Geometry check sheet. Reference: the model listing, model coordinates, mm. Give positions to 0.01 mm unless a question says otherwise; leave off trailing zeros. Loops run counter-clockwise (first coordinate to the right, second up) from the corner with the lowest first, then second, coordinate; pieces in that order, holes last. Notation, with made-up numbers: (-3, 73.5) -> (44, 73.5) arc R21 cw to (44, 91.5) -> close; hole circle Ø1 at (8, 74). An arc over 180 degrees is marked (long way). One line per item, written item: value. Start each with the question number.
(1) Draft check along Y on faces 1 (the face through (-0.59, 4.46, -36.11)), 2 (the face through (0, -2, -35.5)), 3 (the face through (-0.37, -1.66, -36.11)). Enter one of: pulls with the +Y half, pulls with the -Y half, needs draft (parallel to the pull), parting line crosses it, or undercut.
(2) Sectioned sample at A-A, the plane y = 0. Record the cut outline in (x, z), then the cut area to 3 significant figures.
(3) Sectioned sample at C-C, the plane z = -36.1. Record the cut outline in (x, y).
(4) Gauge pin test, flat end, axial feed: pin 1 Ø2.5 at (x, y) = (0, 0) entering from -Z. Record the tip position at first contact, or that the pin passes through.
(5) Scan lines: line 1 along Y through (x, z) = (0, -36.35); line 2 along X through (y, z) = (-1, -35.85); line 3 along Y through (x, z) = (-1.5, -35.65). Record each from-to range of solid material in increasing order. Write a range as from..to.
(6) Sectioned sample at D-D, the plane x = 2. Record the cut outline in (y, z).
from build123d import *

# Parameters (mm, degrees)
F_0102_CYLINDER_SKETCH_R = 4.5
F_0102_CYLINDER_DEPTH    = 1.2
F_0104_CYLINDER_SKETCH_R = 1.7
F_0104_CYLINDER_DEPTH    = 2


with BuildPart() as part:
    # 0102_cylinder_Sketch → 0102_cylinder (new body)
    with BuildSketch(Plane.XY):
        Circle(F_0102_CYLINDER_SKETCH_R)
    extrude(amount=F_0102_CYLINDER_DEPTH)


with BuildPart() as part_1:
    # 0102_cylinder_Translate: moved
    add(part.part.moved(Location((0, 0, -36.7))))


with BuildPart() as body_2:
    # 0104_cylinder_Sketch → 0104_cylinder (new body)
    with BuildSketch(Plane.XY):
        Circle(F_0104_CYLINDER_SKETCH_R)
    extrude(amount=F_0104_CYLINDER_DEPTH)


with BuildPart() as body_2_1:
    # 0104_cylinder_Translate: moved
    add(body_2.part.moved(Location((0, 0, -37))))


with BuildPart() as part_2:
    add(part_1.part)

    # 0106_sub: cut body 2
    add(body_2_1.part, mode=Mode.SUBTRACT)


solid = part_2.part
Calculated:
1. face 1: parting line crosses it
1. face 2: needs draft
1. face 3: undercut
2. outline: (-4.5, -36.7) -> (-1.7, -36.7) -> (-1.7, -35.5) -> (-4.5, -35.5) -> close; (1.7, -36.7) -> (4.5, -36.7) -> (4.5, -35.5) -> (1.7, -35.5) -> close
2. area: 6.72 mm2
3. outline: circle Ø9 at (0, 0); hole circle Ø3.4 at (0, 0)
4. pin 1: passes through
5. line 1: y = -4.5..-1.7, 1.7..4.5
5. line 2: x = -4.39..-1.37, 1.37..4.39
5. line 3: y = -4.24..-0.8, 0.8..4.24
6. outline: (-4.03, -36.7) -> (4.03, -36.7) -> (4.03, -35.5) -> (-4.03, -35.5) -> close
